Build history of the part. All positions in model axes, mm. A direction names the side the tool comes from. Round coordinates to 2 decimals unless told otherwise and drop trailing zeros. Write each loop counter-clockwise with the first axis right and the second up, starting at its lowest first coordinate (ties: lowest second). Pieces come first, ordered by that corner, then holes. Notation, with made-up numbers: (-10, -29.5) - (35, -29.5) arc R17 cw to (35, -0.5) - close; hole circle Ø5 at (8, 65). An arc over 180 degrees is marked (long way). Answer as a JSON object with one key per item and string values. Group by question number.
Item 1: Slice it at B-B, the plane y = 1. Give the number of separate pieces and of enclosed holes in the cut face, then the cut area to 3 significant figures.
Item 2: Probe line 1 (Z direction, x = -68, y = 0.6); line 2 (Z direction, x = 106.5, y = 2.6); line 3 (X direction, y = 0.8, z = 14). List the from-to ranges inside material, lowest first. Write a range as from..to.
Item 3: Which spindle directions (+Z, -Z, +X, -X, +Y, -Y) get a long thin tool onto all of the face, cutting with end or side? Do faces 1 (the flat face through (-2, 3, 0)), 2 (the flat face through (-47.48, 1.52, 7.2)). Say none if no direction does.
Item 4: Flat gauge pin, fed straight in: pin 1 (2.5 mm diameter, centred on x = 21.5, z = -15, fed in from +Y). Where does the tip first touch, or does it go through?
Item 5: Two-plate mould, pull along Z, no slides. Class faces 3 (the flat face through (47.19, 1.521, -7.354)), 4 (the flat face through (-2, 0, 0)): +Z half, -Z half, draft (parallel to the pull), parting line (faces both ways), or undercut.
Item 6: Slice it at A-A, the plane x = 61. List the corners of the cut face in (y, z), then the cut area to 3 significant figures.
from build123d import *

# Parameters (mm, degrees)
SKETCH_1_W             = 250
SKETCH_1_H             = 60
EXTRUDE_1_DEPTH        = 3
SKETCH_2_R             = 1.5
CUT_EXTRUDE_1_DEPTH    = 129.5846025
SKETCH_3_R             = 1.6
CUT_EXTRUDE_2_DEPTH    = 129.5846025
SKETCH_4_R             = 1.6
CUT_EXTRUDE_3_DEPTH    = 129.5846025
FILLET_1_R             = 2
CUT_EXTRUDE_4_DEPTH    = 129.5846025
FILLET_2_R             = 2
FILLET_2_OF_MIRROR_1_R = 2
CUT_EXTRUDE_5_DEPTH    = 129.5846025
FILLET_3_R             = 1


with BuildPart() as part:
    # 草图1 → 凸台-拉伸1 (new body)
    with BuildSketch(Plane(origin=(0, 0, 0), x_dir=(1, 0, 0), z_dir=(0, 1, 0))):
        Rectangle(SKETCH_1_W, SKETCH_1_H)
    extrude(amount=EXTRUDE_1_DEPTH)

    # 草图2 → 切除-拉伸1 (cut, through all)
    with BuildSketch(Plane(origin=(0, 3, 0), x_dir=(1, 0, 0), z_dir=(0, 1, 0))):
        with Locations(Location((0, -26.6, 0), (0, 0, 270))):
            Circle(SKETCH_2_R)
        with Locations(Location((10, -2.9, 0), (0, 0, 270))):
            Circle(SKETCH_2_R)
        with Locations(Location((-10, -2.9, 0), (0, 0, 270))):
            Circle(SKETCH_2_R)
    extrude(amount=-CUT_EXTRUDE_1_DEPTH, mode=Mode.SUBTRACT)

    # 草图3 → 切除-拉伸2 (cut, through all)
    with BuildSketch(Plane.XZ):
        with Locations(Location((122, 15, 0), (0, 0, 270))):
            Circle(SKETCH_3_R)
        with Locations(Location((122, -5, 0), (0, 0, 270))):
            Circle(SKETCH_3_R)
        with Locations(Location((-122, 15, 0), (0, 0, 270))):
            Circle(SKETCH_3_R)
        with Locations(Location((-122, -5, 0), (0, 0, 270))):
            Circle(SKETCH_3_R)
    extrude(amount=-CUT_EXTRUDE_2_DEPTH, mode=Mode.SUBTRACT)

    # 草图4 → 切除-拉伸3 (cut, through all)
    with BuildSketch(Plane(origin=(0, 3, 0), x_dir=(1, 0, 0), z_dir=(0, 1, 0))):
        with Locations(Location((-21.5, -5, 0), (0, 0, 270))):
            Circle(SKETCH_4_R)
        with Locations(Location((-21.5, 15, 0), (0, 0, 270))):
            Circle(SKETCH_4_R)
        with Locations(Location((21.5, -5, 0), (0, 0, 270))):
            Circle(SKETCH_4_R)
        with Locations(Location((21.5, 15, 0), (0, 0, 270))):
            Circle(SKETCH_4_R)
    extrude(amount=-CUT_EXTRUDE_3_DEPTH, mode=Mode.SUBTRACT)

    # 圆角1
    fillet_1_edges = [part.edges().sort_by_distance(p)[0] for p in [
        (125, 1.5, 30),
        (-125, 1.5, 30),
        (-125, 1.5, -30),
        (125, 1.5, -30),
    ]]
    fillet(fillet_1_edges, radius=FILLET_1_R)

    # 草图5 → 切除-拉伸4 (cut, through all)
    with BuildSketch(Plane(origin=(0, 3, 0), x_dir=(1, 0, 0), z_dir=(0, 1, 0))):
        Polygon((-44.680187557, 20), (-98.819812443, 20), (-71.75, 5.658377514), align=None)
        Polygon((-34, -14.341622486), (-34, 14.341622486), (-61.069812443, 0), align=None)
        Polygon((-71.75, -5.658377514), (-98.819812443, -20), (-44.680187557, -20), align=None)
        Polygon((-82.430187557, 0), (-109.5, 14.341622486), (-109.5, -14.341622486), align=None)
    cut_extrude_4 = extrude(amount=-CUT_EXTRUDE_4_DEPTH, mode=Mode.SUBTRACT)

    # 圆角2
    fillet_2_edges = [part.edges().sort_by_distance(p)[0] for p in [
        (-71.75, 1.5, 5.658377514),
        (-44.680187557, 1.5, 20),
        (-98.819812443, 1.5, 20),
        (-61.069812443, 1.5, 0),
        (-34, 1.5, -14.341622486),
        (-34, 1.5, 14.341622486),
        (-109.5, 1.5, -14.341622486),
        (-82.430187557, 1.5, 0),
        (-109.5, 1.5, 14.341622486),
        (-98.819812443, 1.5, -20),
        (-44.680187557, 1.5, -20),
        (-71.75, 1.5, -5.658377514),
    ]]
    fillet(fillet_2_edges, radius=FILLET_2_R)

    # 镜向1: 切除-拉伸4 across plane
    add(cut_extrude_4.mirror(Plane.ZY), mode=Mode.SUBTRACT)

    # 圆角2 of 镜向1
    fillet_2_of_mirror_1_edges = [part.edges().sort_by_distance(p)[0] for p in [
        (71.75, 1.5, 5.658377514),
        (44.680187557, 1.5, 20),
        (98.819812443, 1.5, 20),
        (61.069812443, 1.5, 0),
        (34, 1.5, -14.341622486),
        (34, 1.5, 14.341622486),
        (109.5, 1.5, -14.341622486),
        (82.430187557, 1.5, 0),
        (109.5, 1.5, 14.341622486),
        (98.819812443, 1.5, -20),
        (44.680187557, 1.5, -20),
        (71.75, 1.5, -5.658377514),
    ]]
    fillet(fillet_2_of_mirror_1_edges, radius=FILLET_2_OF_MIRROR_1_R)

    # 草图6 → 切除-拉伸5 (cut, through all)
    with BuildSketch(Plane(origin=(0, 3, 0), x_dir=(1, 0, 0), z_dir=(0, 1, 0))):
        Polygon((0, 5.452994616), (10, 22.773502692), (-10, 22.773502692), align=None)
    extrude(amount=-CUT_EXTRUDE_5_DEPTH, mode=Mode.SUBTRACT)

    # 圆角3
    fillet_3_edges = [part.edges().sort_by_distance(p)[0] for p in [
        (0, 1.5, -5.452994616),
        (-10, 1.5, -22.773502692),
        (10, 1.5, -22.773502692),
    ]]
    fillet(fillet_3_edges, radius=FILLET_3_R)


solid = part.part
Geometry says:
{
 "1": {"separate pieces": "1", "enclosed holes": "20", "area": "11,800 mm^2"},
 "2": {"line 1": "z = -30..-20, -7.65..7.65, 20..30", "line 2": "z = -30..-12.75, 12.75..30", "line 3": "x = -125..-123.25, -120.75..-87.49, -56.01..56.01, 87.49..120.75, 123.25..125"},
 "3": {"face 1": "+Z, -Z, +X, -X, +Y", "face 2": "+Y, -Y"},
 "4": {"pin 1": "passes through"},
 "5": {"face 3": "undercut", "face 4": "draft"},
 "6": {"outline": "(0, -30) - (3, -30) - (3, -20) - (0, -20) - close; (0, -11.35) - (3, -11.35) - (3, 11.35) - (0, 11.35) - close; (0, 20) - (3, 20) - (3, 30) - (0, 30) - close", "area": "128 mm^2"}
}
